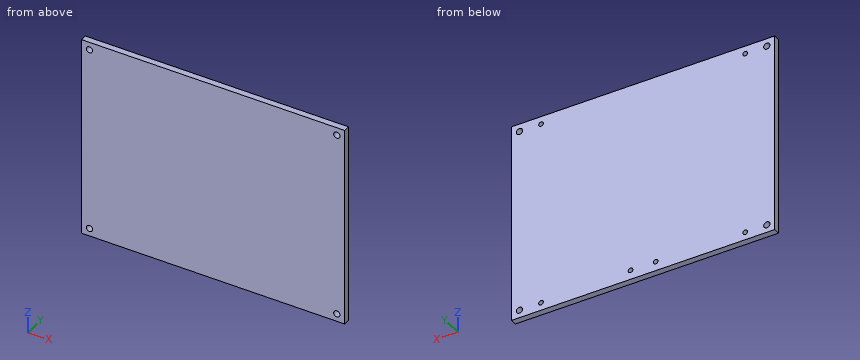
from build123d import *

# Parameters (mm, degrees)
SKETCH1_W           = 167.5
SKETCH1_H           = 130
BOSS_EXTRUDE1_DEPTH = 4
SKETCH2_R           = 1.5
CUT_EXTRUDE1_DEPTH  = 3
SKETCH3_R           = 1.5
CUT_EXTRUDE2_DEPTH  = 3
SKETCH5_R           = 2
CUT_EXTRUDE3_DEPTH  = 10


with BuildPart() as part:
    # Sketch1 → Boss-Extrude1 (new body)
    with BuildSketch(Plane(origin=(0, 0, 0), x_dir=(1, 0, 0), z_dir=(0, 1, 0))):
        Rectangle(SKETCH1_W, SKETCH1_H)
    extrude(amount=BOSS_EXTRUDE1_DEPTH)

    # Sketch2 → Cut-Extrude1 (cut)
    with BuildSketch(Plane(origin=(0, 4, 0), x_dir=(1, 0, 0), z_dir=(0, 1, 0))):
        with Locations(Location((-65, -60, 0), (0, 0, 270))):
            Circle(SKETCH2_R)
        with Locations(Location((65, -60, 0), (0, 0, 270))):
            Circle(SKETCH2_R)
        with Locations(Location((65, 60, 0), (0, 0, 270))):
            Circle(SKETCH2_R)
        with Locations(Location((-65, 60, 0), (0, 0, 270))):
            Circle(SKETCH2_R)
    extrude(amount=-CUT_EXTRUDE1_DEPTH, mode=Mode.SUBTRACT)

    # Sketch3 → Cut-Extrude2 (cut)
    with BuildSketch(Plane(origin=(0, 4, 0), x_dir=(1, 0, 0), z_dir=(0, 1, 0))):
        with Locations(Location((-8, 59, 0), (0, 0, 270))):
            Circle(SKETCH3_R)
        with Locations(Location((8, 59, 0), (0, 0, 270))):
            Circle(SKETCH3_R)
    extrude(amount=-CUT_EXTRUDE2_DEPTH, mode=Mode.SUBTRACT)

    # Sketch5 → Cut-Extrude3 (cut)
    with BuildSketch(Plane(origin=(0, 4, 0), x_dir=(1, 0, 0), z_dir=(0, 1, 0))):
        with Locations(Location((-78.75, 60, 0), (0, 0, 270))):
            Circle(SKETCH5_R)
        with Locations(Location((78.75, 60, 0), (0, 0, 270))):
            Circle(SKETCH5_R)
        with Locations(Location((78.75, -60, 0), (0, 0, 270))):
            Circle(SKETCH5_R)
        with Locations(Location((-78.75, -60, 0), (0, 0, 270))):
            Circle(SKETCH5_R)
    extrude(amount=-CUT_EXTRUDE3_DEPTH, mode=Mode.SUBTRACT)


solid = part.part
Model file for the job. Use its own axes, mm. Round coordinates to 2 decimals unless told otherwise and drop trailing zeros. Loops run counter-clockwise (first coordinate to the right, second up) from the corner with the lowest first, then second, coordinate; pieces in that order, holes last.
1. Band-saw the part on A-A, the plane x = -78.75. List the corners of the cut face in (y, z).
Check values:
outline: (0, -65) - (4, -65) - (4, -62) - (0, -62) - close; (0, -58) - (4, -58) - (4, 58) - (0, 58) - close; (0, 62) - (4, 62) - (4, 65) - (0, 65) - close
2. Drop flat-ended pins along their axis: P1, Ø2.5, axis at x = 65, z = -60, coming from the +Y side; P2, Ø2.5, axis at x = 78.75, z = -60, coming from the -Y side. Give the stop position or say it passes through.
Check values:
P1: stops at y = 1
P2: passes through
3. Wall check: probe 1 along Z at (x, y) = (-65, 2.5); probe 2 along X at (y, z) = (3.3, 60). Give the ranges that are in metal, low to high.
Check values:
probe 1: z = -65 to -61.5, -58.5 to 58.5, 61.5 to 65
probe 2: x = -83.75 to -80.75, -76.75 to -66.5, -63.5 to 63.5, 66.5 to 76.75, 80.75 to 83.75
